Here's how the part is built. I have some questions about the finished solid (model axes, mm). Give positions to 0.01 mm unless a question says otherwise; leave off trailing zeros. Write each loop counter-clockwise with the first axis right and the second up, starting at its lowest first coordinate (ties: lowest second). Pieces come first, ordered by that corner, then holes. Notation, with made-up numbers: (-16.75, 14) - (26.25, 14) arc R32 ccw to (26.25, 45) - close; hole circle Ø2 at (-29.75, 85.25). An arc over 180 degrees is marked (long way). Use a Markdown table: item, result.
Autodesk Inventor part; units mm, degrees
ref_plane "YZ Plane" through (0, 0, 0) normal (1, 0, 0) x (0, 1, 0)
ref_plane "XZ Plane" through (0, 0, 0) normal (0, 1, 0) x (-1, 0, 0)
ref_plane "XY Plane" through (0, 0, 0) normal (0, 0, 1) x (1, 0, 0)
sketch "スケッチ1" plane through (0, 0, 0) normal (1, 0, 0) x (0, 1, 0)
  line L0 (0, 0) -> (-5, 0)
  line L1 (-5, 0) -> (-5, -30)
  line L2 (-5, -30) -> (0, -30)
  line L3 (0, -30) -> (0, 0)
  dimension "d0" = 30
  dimension "d1" = 5
extrude "押し出し1" add sketch "スケッチ1" along normal blind 280
sketch "スケッチ2" plane through (0, -5, -30) normal (0, -1, 0) x (1, 0, 0)
  line L0 (280, 30) -> (280, 0)
  line L1 (0, 0) -> (280, 0)
  point P0 (0, 30)
  point P1 (269, 13)
  dimension "d4" = 11
  dimension "d12" = 13
hole "穴1" at (269, -5, -17) direction (0, 1, 0) diameter 11 end through all
sketch "スケッチ4" plane through (280, 0, -30) normal (0, 0, -1) x (-1, 0, 0)
  line L0 (280, 0) -> (0, 0)
  line L1 (280, -5) -> (280, 0)
  point P0 (260, -2.5)
  point P1 (40, -2.5)
  dimension "d27" = 2.5
  dimension "d28" = 20
  dimension "d36" = 220
hole "穴3" at (20, -2.5, -30) at (240, -2.5, -30) direction (0, 0, 1) diameter 2.459 end through all
sketch "スケッチ5" plane through (0, -5, -30) normal (0, -1, 0) x (1, 0, 0)
  circle A0 centre (269, 13) radius 5.5
  point P0 (0, 30)
  point P1 (269, 4.5)
  point P2 (277.5, 13)
  point P3 (269, 21.5)
  point P4 (260.5, 13)
  dimension "d39" = 360
  dimension "d41" = 8.5
hole "穴4" at (269, -5, -25.5) at (277.5, -5, -17) at (269, -5, -8.5) at (260.5, -5, -17) direction (0, 1, 0) diameter 3 end through all
properties part number "横長2ndフラットバー" material "アルミニウム 6061"
Item 1: Will this pin go through, and if not, where does the flat tip stop? pin 1 Ø1.8 at (x, z) = (269, -8.5) entering from -Y.
Values:
| item | result |
|---|---|
| pin 1 | passes through |
Item 2: I need wall thicknesses on line 1 along X through (y, z) = (-2.2, -8.5); line 2 along X through (y, z) = (-2.5, -11); line 3 along Z through (x, y) = (269, -2.25). Which ranges of each line are inside material? Lowest first, please. Write a range as [from, to].
Values:
| item | result |
|---|---|
| line 1 | x = [0, 18.81], [21.19, 238.81], [241.19, 267.5], [270.5, 280] |
| line 2 | x = [0, 18.77], [21.23, 238.77], [241.23, 280] |
| line 3 | z = [-30, -27], [-24, -22.5], [-11.5, -10], [-7, 0] |
Item 3: Thinking about a two-plate mould opening in X: for faces 1 (the cylindrical face through (274.37, -2.46, -15.81)), 2 (the flat face through (138, 0, -15)), 3 (the flat face through (280, -3, -15)), 4 (the flat face through (0, -3, -15)), which applies, +X half, -X half, draft (parallel to the pull), parting line (faces both ways), or undercut?
Values:
| item | result |
|---|---|
| face 1 | undercut |
| face 2 | draft |
| face 3 | +X half |
| face 4 | -X half |
Item 4: If we section it at A-A, the plane y = -2.5: Write out the boundary of the cut face in (x, z).
Values:
| item | result |
|---|---|
| outline | (0, -30) - (18.77, -30) - (18.77, 0) - (0, 0) - close; (21.23, -30) - (238.77, -30) - (238.77, 0) - (21.23, 0) - close; (241.23, -30) - (280, -30) - (280, 0) - (241.23, 0) - close; hole circle Ø3 at (260.5, -17); hole circle Ø11 at (269, -17); hole circle Ø3 at (269, -25.5); hole circle Ø3 at (269, -8.5); hole circle Ø3 at (277.5, -17) |
